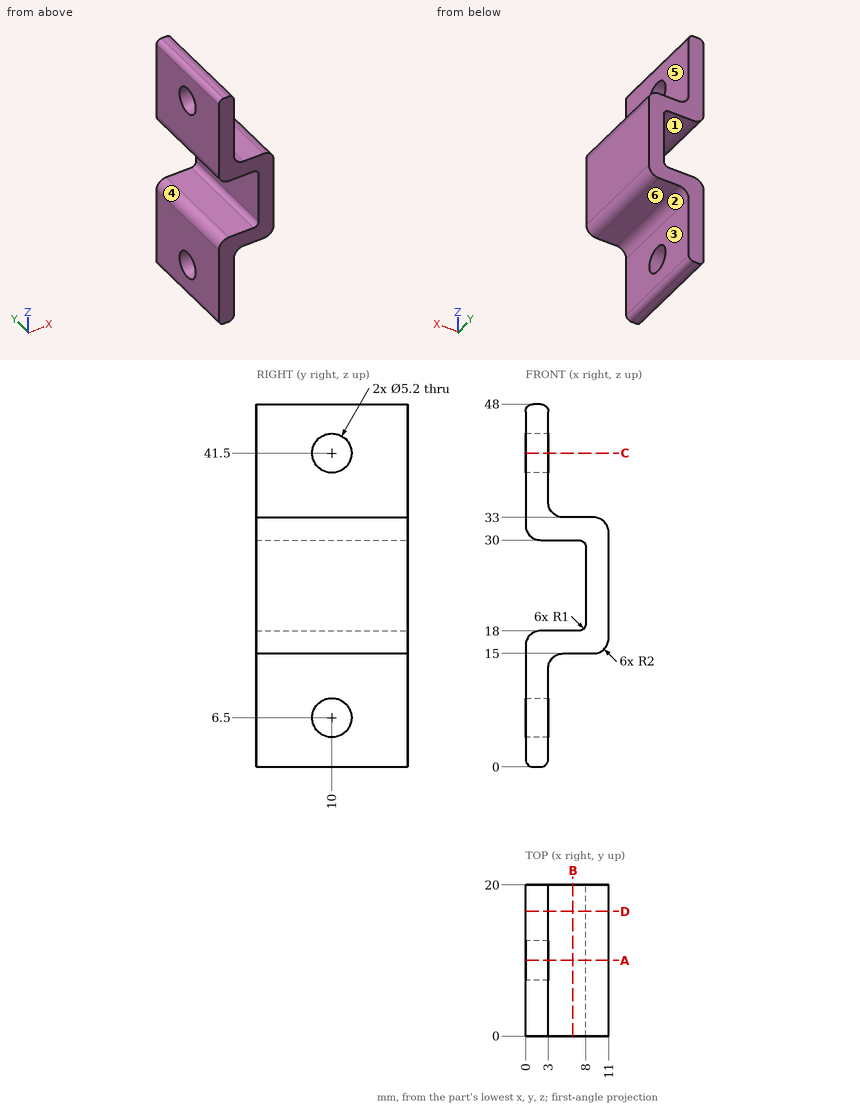
Part print with two shaded views. Sizes in mm from the minimum x, y, z corner. A direction names the side the tool comes from. Round coordinates to 2 decimals unless told otherwise and drop trailing zeros. Write each loop counter-clockwise with the first axis right and the second up, starting at its lowest first coordinate (ties: lowest second). Pieces come first, ordered by that corner, then holes. Notation, with made-up numbers: M 21.25,83 L 45.25,83 A38 ccw 45.25,121 Z; hole C 35,89.5 d10. An arc over 180 degrees is marked long. Answer as CSV lines item,"result". Start each with the question number.
1) Which spindle directions (+Z, -Z, +X, -X, +Y, -Y) get a long thin tool onto all of the face, cutting with end or side? Do the marked faces 4, 5 and 6. Say none if no direction does.
2) Drill centre lines: L1, parallel to Y at x = 0.75, z = 41.5; L2, parallel to Z at x = 6.75, y = 4.25; L3, parallel to Z at x = 2.25, y = 8.75. Where is each one in solid material? Low to high.
3) Mould opens along Z. For the marked faces 1, 2 and 3 say: +Z half, -Z half, draft (parallel to the pull), parting line (faces both ways), or undercut.
4) Band-saw the part on A-A (y = 10). Count the separate pieces of the cut face and the enclosed holes in it, then the cut area to 3 significant figures.
5) Band-saw the part on C-C (z = 41.5). List the corners of the cut face in (x, y), then the cut area to 3 significant figures.
6) Band-saw the part on B-B (x = 6.25). List the corners of the cut face in (y, z).
7) Drop flat-ended pins along their axis: pin 1 (7 mm diameter, centred on y = 10, z = 41.5, fed in from -X); pin 2 (4 mm diameter, centred on y = 15.5, z = 20.5, fed in from -X); pin 3 (3 mm diameter, centred on y = 7, z = 24.5, fed in from -X); pin 4 (6 mm diameter, centred on y = 14, z = 39, fed in from +X). Give the stop position or say it passes through.
8) Band-saw the part on D-D (y = 16.5). List the corners of the cut face in (x, z).
Worked out:
1,face 4,"-X, +Y, -Y"
1,face 5,"+Z, +X, +Y, -Y"
1,face 6,"-Z, +X, +Y, -Y"
2,L1,"0 to 7.4, 12.6 to 20"
2,L2,"15 to 18, 30 to 33"
2,L3,"0.03 to 4.22, 8.78 to 18, 30 to 39.22, 43.78 to 47.97"
3,face 1,"undercut"
3,face 2,"-Z half"
3,face 3,"draft"
4,separate pieces,"3"
4,enclosed holes,"0"
4,area,"159 mm²"
5,outline,"M 0,0 L 3,0 L 3,7.4 L 0,7.4 Z; M 0,12.6 L 3,12.6 L 3,20 L 0,20 Z"
5,area,"44.4 mm²"
6,outline,"M 0,15 L 20,15 L 20,18 L 0,18 Z; M 0,30 L 20,30 L 20,33 L 0,33 Z"
7,pin 1,"x = 0"
7,pin 2,"x = 7.87"
7,pin 3,"x = 8"
7,pin 4,"x = 3"
8,outline,"M 0,1 A1 ccw 1,0 L 2,0 A1 ccw 3,1 L 3,13 A2 cw 5,15 L 9,15 A2 ccw 11,17 L 11,31 A2 ccw 9,33 L 5,33 A2 cw 3,35 L 3,47 A1 ccw 2,48 L 1,48 A1 ccw 0,47 L 0,32 A2 ccw 2,30 L 7,30 A1 cw 8,29 L 8,19 A1 cw 7,18 L 2,18 A2 ccw 0,16 Z"
